from build123d import *

# Parameters (mm, degrees)
F0_W     = 25.4
F0_H     = 254
F1_DEPTH = 25.4
F2_DEPTH = 127
F4_D     = 5.1054


with BuildPart() as f1:
    # F0 (on Top) → F1 (new body)
    with BuildSketch(Plane.XY):
        with Locations((-43.66958, 89.766972)):
            Rectangle(F0_W, F0_H)
    extrude(amount=F1_DEPTH)

    # F0 (on Top) → F2 (join)
    with BuildSketch(Plane.XY):
        Polygon((-30.96958, -37.233028), (-56.36958, -37.233028), (-56.36958, -88.033028), align=None)
    extrude(amount=F2_DEPTH)

    # F4 (through all)
    with Locations(Plane.XY.offset(25.4)):
        with Locations((-43.66958, 204.066972), (-43.66958, 153.266972), (-43.66958, 178.666972), (-43.66958, 127.866972), (-43.66958, 102.466972), (-43.66958, 77.066972), (-43.66958, 0.866972), (-43.66958, 51.666972), (-43.66958, 26.266972), (-43.66958, -24.533028)):
            Hole(F4_D / 2)


solid = f1.part
Source: CAD feature listing. Evaluate the final solid. Frame: model axes, mm. A direction names the side the tool comes from. Round coordinates to 2 decimals unless told otherwise and drop trailing zeros. Order: outer loops, then holes, each group sorted by start corner. A loop starts at its lowest first (then second) coordinate and runs counter-clockwise, first axis right, second up. Notation, with made-up numbers: (48, 10) - (107, 10) arc R5 cw to (107, 17) - close; hole circle Ø5 at (-17.5, 57.5). An arc over 180 degrees is marked (long way). Use a Markdown table: item, result. Add a question column.
1. Section query D-D (x = -35.75). Return the cut outline in (y, z).
2. First-contact query: pin 1 (3 mm diameter, centred on x = -53, z = 111, fed in from +Y); pin 2 (6.5 mm diameter, centred on x = -43.67, y = 204.07, fed in from +Z). Flat tips, straight axial feed; report the tip coordinate or a pass-through.
3. Section query A-A (x = -52.75). Return the cut outline in (y, z).
4. Line query: probe 1 along Z at (x, y) = (-52.25, 111); probe 2 along Y at (x, z) = (-40.25, 72); probe 3 along Y at (x, z) = (-54.75, 95.5). Output: solid intervals per line, ascending.
5. Section query B-B (y = 65.5). Return the cut outline in (x, z).
6. Set-up query: faces 1 (the cylindrical face through (-41.788, 129.592, 12.522)), 2 (the flat face through (-44, 92, 25.4)). Return all of +Z, -Z, +X, -X, +Y, -Y with unobstructed straight access to the full face (end or side cutting, diameter ignored); none if empty.
7. Mould query, pull axis Y, two halves, no side actions, for faces 3 (the flat face through (-56.37, 20, 11)), 4 (the flat face through (-43.85, -62.99, 62.61)), 5 (the cylindrical face through (-43.116, 150.775, 12.522)). Classes: +Y half, -Y half, draft (parallel to the pull), parting line (faces both ways), or undercut.
8. Section query C-C (z = 54). Return the cut outline in (x, y), then the cut area to 3 significant figures.
Derived:
| question | item | result |
|---|---|---|
| 1 | outline | (-46.79, 0) - (216.77, 0) - (216.77, 25.4) - (-37.23, 25.4) - (-37.23, 127) - (-46.79, 127) - close |
| 2 | pin 1 | y = -37.23 |
| 2 | pin 2 | z = 25.4 |
| 3 | outline | (-80.79, 0) - (216.77, 0) - (216.77, 25.4) - (-37.23, 25.4) - (-37.23, 127) - (-80.79, 127) - close |
| 4 | probe 1 | 0 to 25.4 |
| 4 | probe 2 | -55.79 to -37.23 |
| 4 | probe 3 | -84.79 to -37.23 |
| 5 | outline | (-56.37, 0) - (-30.97, 0) - (-30.97, 25.4) - (-56.37, 25.4) - close |
| 6 | face 1 | +Z, -Z |
| 6 | face 2 | +Z, +X, -X, +Y |
| 7 | face 3 | draft |
| 7 | face 4 | -Y half |
| 7 | face 5 | undercut |
| 8 | outline | (-56.37, -88.03) - (-30.97, -37.23) - (-56.37, -37.23) - close |
| 8 | area | 645 mm2 |
